Read the model definition and answer for the solid it produces. Units are mm, in the model's axes. A direction names the side the tool comes from. Coordinates: 2 decimals unless noted, no trailing zeros. Write each loop counter-clockwise with the first axis right and the second up, starting at its lowest first coordinate (ties: lowest second). Pieces come first, ordered by that corner, then holes.
from build123d import *

# Parameters (mm, degrees)
BASE_FLANGE1_DEPTH   = 40
FILLET1_R            = 2
SKETCH6_R            = 1.55
CUT_EXTRUDE1_DEPTH   = 10
M4_CLEARANCE_HOLE1_D = 4.8


# Sheet-metal steps are written as plain solids
with BuildPart() as part:
    # Sketch1 → Base-Flange1 (new body)
    with BuildSketch(Plane.XY):
        with BuildLine():
            Line((-61, 0), (-2, 0))
            ThreePointArc((-2, 0), (-0.585786438, -0.585786438), (0, -2))
            Line((0, -2), (0, -30))
            Line((0, -30), (-1, -30))
            Line((-1, -30), (-1, -2))
            ThreePointArc((-1, -2), (-1.292893219, -1.292893219), (-2, -1))
            Line((-2, -1), (-61, -1))
            Line((-61, -1), (-61, 0))
        make_face()
    extrude(amount=BASE_FLANGE1_DEPTH)

    # Fillet1
    fillet1_edges = [part.edges().sort_by_distance(p)[0] for p in [
        (-61, -0.5, 40),
        (-61, -0.5, 0),
        (-0.5, -30, 40),
        (-0.5, -30, 0),
    ]]
    fillet(fillet1_edges, radius=FILLET1_R)

    # Sketch6 → Cut-Extrude1 (cut)
    with BuildSketch(Plane(origin=(0, 0, 0), x_dir=(1, 0, 0), z_dir=(0, 1, 0))):
        with Locations(Location((-56.3, -4.9, 0), (0, 0, 270))):
            Circle(SKETCH6_R)
        with Locations(Location((-48, -4.9, 0), (0, 0, 270))):
            Circle(SKETCH6_R)
    extrude(amount=-CUT_EXTRUDE1_DEPTH, mode=Mode.SUBTRACT)

    # M4 Clearance Hole1 (through all)
    with Locations(Plane(origin=(0, 0, 0), x_dir=(0, 0, -1), z_dir=(1, 0, 0))):
        with Locations((-35.1, -19.849994255), (-5.1, -19.849994255)):
            Hole(M4_CLEARANCE_HOLE1_D / 2)


solid = part.part
Item 1: For faces 5 (the cylindrical face through (-60.43, -0.49, 0.6)), 6 (the flat face through (-31, -1, 20)), determine the directions among +Z, -Z, +X, -X, +Y, -Y from which every point of the face is accessible in a straight line to the end or side of a thin tool.
Item 2: The part is cut by section B-B (x = -48). Give the vertices of the cut face in (y, z), and give its area (3 significant figures).
Item 3: The part is cut by section A-A (z = 35.1). Give the vertices of the cut face in (x, y), and give its area (3 significant figures).
Item 4: The part is cut by section D-D (z = 4.9). Give the vertices of the cut face in (x, y).
Item 5: Find the intervals of material crossed by probe 1 along X at (y, z) = (-0.5, 4.9); probe 2 along Y at (x, z) = (-12.5, 3), in increasing order.
Item 6: Given pin 1 (1.5 mm diameter, centred on x = -15, z = 32, fed in from -Y); pin 2 (1 mm diameter, centred on y = -9.5, z = 21.5, fed in from -X), each flat-ended and moving along its own axis, determine where each tip first touches the part or whether it passes through.
Item 7: Determine the mould class of faces 1 (the cylindrical face through (-60.43, -0.49, 39.4)), 2 (the cylindrical face through (-0.51, -29.43, 0.6)), 3 (the cylindrical face through (-49.375, -0.493, 5.615)), 4 (the flat face through (-1, -16, 20)) for opening direction Z: +Z half, -Z half, draft (parallel to the pull), parting line (faces both ways), or undercut.
Item 8: The part is cut by section C-C (y = -21.5). Give the vertices of the cut face in (x, z), and give its area (3 significant figures).
Answer:
1. face 5: -Z, -X, +Y, -Y
1. face 6: +Z, -Z, -X, -Y
2. outline: (-1, 0) - (0, 0) - (0, 3.35) - (-1, 3.35) - close; (-1, 6.45) - (0, 6.45) - (0, 40) - (-1, 40) - close
2. area: 36.9 mm2
3. outline: (-61, -1) - (-2, -1) arc R1 cw to (-1, -2) - (-1, -17.45) - (0, -17.45) - (0, -2) arc R2 ccw to (-2, 0) - (-61, 0) - close; (-1, -30) - (0, -30) - (0, -22.25) - (-1, -22.25) - close
3. area: 84.6 mm2
4. outline: (-61, -1) - (-57.85, -1) - (-57.85, 0) - (-61, 0) - close; (-54.75, -1) - (-49.55, -1) - (-49.55, 0) - (-54.75, 0) - close; (-46.45, -1) - (-2, -1) arc R1 cw to (-1, -2) - (-1, -17.46) - (0, -17.46) - (0, -2) arc R2 ccw to (-2, 0) - (-46.45, 0) - close; (-1, -30) - (0, -30) - (0, -22.24) - (-1, -22.24) - close
5. probe 1: x = -61 to -57.85, -54.75 to -49.55, -46.45 to -0.68
5. probe 2: y = -1 to 0
6. pin 1: stops at y = -1
6. pin 2: stops at x = -1
7. face 1: +Z half
7. face 2: -Z half
7. face 3: undercut
7. face 4: draft
8. outline: (-1, 0) - (0, 0) - (0, 3.36) - (-1, 3.36) - close; (-1, 6.84) - (0, 6.84) - (0, 33.36) - (-1, 33.36) - close; (-1, 36.84) - (0, 36.84) - (0, 40) - (-1, 40) - close
8. area: 33.0 mm2
